The listing builds one solid part. Answer for the finished solid, in the listing's coordinates (mm). A direction names the side the tool comes from. Coordinates: 2 decimals unless noted, no trailing zeros. Write each loop counter-clockwise with the first axis right and the second up, starting at its lowest first coordinate (ties: lowest second). Pieces come first, ordered by that corner, then holes.
from build123d import *

# Parameters (mm, degrees)
SKETCH107_W         = 48
SKETCH107_H         = 56
PAD026_DEPTH        = 2
SKETCH108_R         = 1.75
HOLE046_DEPTH       = 25
SKETCH109_W         = 48
SKETCH109_H         = 32
PAD027_DEPTH        = 30
SKETCH110_W         = 40.4
SKETCH110_H         = 24.4
POCKET033_DEPTH     = 30
SKETCH111_W         = 20
SKETCH111_H         = 20
SKETCH111_W_2       = 40
POCKET034_DEPTH     = 28
SKETCH112_W         = 24
SKETCH112_H         = 22
POCKET035_DEPTH     = 50
SKETCH113_R         = 1.75
HOLE047_DEPTH       = 25
HOLE048_D           = 3.5
HOLE048_DEPTH       = 25
HOLE048_CSINK_D     = 8
HOLE048_CSINK_ANGLE = 90
HOLE048_TIPS_R      = 1.75
FILLET037_R         = 1
PAD_DEPTH           = 14
SKETCH115_R         = 4
HOLE_DEPTH          = 25
HOLE_TIPS_R         = 4
FILLET_R            = 1
FILLET038_R         = 1
FILLET039_R         = 1


with BuildPart() as part:
    # Sketch107 → Pad026 (new body)
    with BuildSketch(Plane.XY):
        Rectangle(SKETCH107_W, SKETCH107_H)
    extrude(amount=PAD026_DEPTH)

    # Sketch108 (on Face6 of Pad026) → Hole046 (cut)
    with BuildSketch(Plane.XY.offset(2)):
        with Locations((18, 22)):
            Circle(SKETCH108_R)
        with Locations((18, -22)):
            Circle(SKETCH108_R)
    hole046 = extrude(amount=-HOLE046_DEPTH, mode=Mode.SUBTRACT)

    # Mirrored041: Hole046 across Sketch108 V_Axis
    add(hole046.mirror(Plane(origin=(0, 0, 2), x_dir=(0, 0, 1), z_dir=(1, 0, 0))), mode=Mode.SUBTRACT)

    # Sketch109 (on Face5 of Mirrored041) → Pad027 (join)
    with BuildSketch(Plane.XY.offset(2)):
        Rectangle(SKETCH109_W, SKETCH109_H)
    extrude(amount=PAD027_DEPTH)

    # Sketch110 (on Face12 of Pad027) → Pocket033 (cut)
    with BuildSketch(Plane.XY.offset(32)):
        Rectangle(SKETCH110_W, SKETCH110_H)
    extrude(amount=-POCKET033_DEPTH, mode=Mode.SUBTRACT)

    # Sketch111 (on Face8 of Pocket033) → Pocket034 (cut)
    with BuildSketch(Plane.XY.offset(32)):
        with Locations((0, 10)):
            Rectangle(SKETCH111_W, SKETCH111_H)
        with Locations((20, 0)):
            Rectangle(SKETCH111_W_2, SKETCH111_H)
    extrude(amount=-POCKET034_DEPTH, mode=Mode.SUBTRACT)

    # Sketch112 (on Face3 of Pocket034) → Pocket035 (cut)
    with BuildSketch(Plane(origin=(-24, 0, 0), x_dir=(0, -1, 0), z_dir=(-1, 0, 0))):
        with Locations((0, 14)):
            Rectangle(SKETCH112_W, SKETCH112_H)
    extrude(amount=-POCKET035_DEPTH, mode=Mode.SUBTRACT)

    # Sketch113 (on Face34 of Pocket035) → Hole047 (cut)
    with BuildSketch(Plane.XY.offset(2)):
        with Locations((-16.2, 8.2)):
            Circle(SKETCH113_R)
        with Locations((-16.2, -8.2)):
            Circle(SKETCH113_R)
    extrude(amount=-HOLE047_DEPTH, mode=Mode.SUBTRACT)

    # Hole048
    with Locations(Plane(origin=(0, 0, 0), x_dir=(1, 0, 0), z_dir=(0, 0, -1))):
        with Locations((-16.2, -8.2), (-16.2, 8.2)):
            CounterSinkHole(HOLE048_D / 2, HOLE048_CSINK_D / 2, depth=HOLE048_DEPTH, counter_sink_angle=HOLE048_CSINK_ANGLE)

    # Hole048 tips → Hole048 tip 1 section 0
    with BuildSketch(Plane(origin=(0, 0, 25), x_dir=(1, 0, 0), z_dir=(0, 0, -1)), mode=Mode.PRIVATE) as hole048_tip_1_s0:
        with Locations((-16.2, -8.2)):
            Circle(HOLE048_TIPS_R)
    loft([hole048_tip_1_s0.sketch, Vertex(-16.2, 8.2, 26.051506)], mode=Mode.SUBTRACT)

    # Hole048 tips → Hole048 tip 2 section 0
    with BuildSketch(Plane(origin=(0, 0, 25), x_dir=(1, 0, 0), z_dir=(0, 0, -1)), mode=Mode.PRIVATE) as hole048_tip_2_s0:
        with Locations((-16.2, 8.2)):
            Circle(HOLE048_TIPS_R)
    loft([hole048_tip_2_s0.sketch, Vertex(-16.2, -8.2, 26.051506)], mode=Mode.SUBTRACT)

    # Fillet037
    fillet037_edges = [part.edges().sort_by_distance(p)[0] for p in [
        (24, -28, 1),
        (24, 28, 1),
        (-24, -28, 1),
        (-24, 28, 1),
    ]]
    fillet(fillet037_edges, radius=FILLET037_R)

    # Sketch (on Face10 of Fillet037) → Pad (join)
    with BuildSketch(Plane.YZ.offset(24)):
        with BuildLine():
            ThreePointArc((16, 12.999996), (19.221827, 5.221824), (27, 2))
            Line((16, 2), (27, 2))
            Line((16, 12.999996), (16, 2))
        make_face()
    pad = extrude(amount=-PAD_DEPTH)

    # Mirrored: Pad across Sketch V_Axis
    add(pad.mirror(Plane(origin=(24, 0, 0), x_dir=(1, 0, 0), z_dir=(0, 1, 0))))

    # Sketch115 (on Face5 of Pad) → Hole (cut)
    with BuildSketch(Plane.XY.offset(2)):
        with Locations((18, 22)):
            Circle(SKETCH115_R)
        with Locations((18, -22)):
            Circle(SKETCH115_R)
    extrude(amount=HOLE_DEPTH, mode=Mode.SUBTRACT)

    # Hole tips → Hole tip 1 section 0
    with BuildSketch(Plane.XY.offset(27), mode=Mode.PRIVATE) as hole_tip_1_s0:
        with Locations((18, 22)):
            Circle(HOLE_TIPS_R)
    loft([hole_tip_1_s0.sketch, Vertex(18, 22, 29.403442)], mode=Mode.SUBTRACT)

    # Hole tips → Hole tip 2 section 0
    with BuildSketch(Plane.XY.offset(27), mode=Mode.PRIVATE) as hole_tip_2_s0:
        with Locations((18, -22)):
            Circle(HOLE_TIPS_R)
    loft([hole_tip_2_s0.sketch, Vertex(18, -22, 29.403442)], mode=Mode.SUBTRACT)

    # Fillet
    fillet_edges = [part.edges().sort_by_distance(p)[0] for p in [
        (-24, -16, 17),
        (-24, 16, 17),
    ]]
    fillet(fillet_edges, radius=FILLET_R)

    # Fillet038
    fillet038_edges = [part.edges().sort_by_distance(p)[0] for p in [
        (20.2, 10, 28.5),
        (20.2, -10, 28.5),
    ]]
    fillet(fillet038_edges, radius=FILLET038_R)

    # Fillet039
    fillet039_edges = [part.edges().sort_by_distance(p)[0] for p in [
        (24, 10, 28.5),
        (24, -10, 28.5),
    ]]
    fillet(fillet039_edges, radius=FILLET039_R)


solid = part.part
1. Section B-B on y = 8.2 is taken. Give the vertices of the cut face in (x, z).
Results found:
outline: (-24, 0) - (-20.2, 0) - (-18.2, 2) - (-20.2, 2) - (-20.2, 3) - (-24, 3) - close; (-24, 25) - (-20.2, 25) - (-20.2, 32) - (-24, 32) - close; (-14.2, 2) - (-12.2, 0) - (24, 0) - (24, 3) - (20.2, 3) - (20.2, 2) - close
2. Find the intervals of material crossed by L1, parallel to Y at x = 18, z = 0.9; L2, parallel to Y at x = -18.5, z = 18; L3, parallel to X at y = 15, z = 28.5, in increasing order.
Results found:
L1: y = -28 to -23.75, -20.25 to 20.25, 23.75 to 28
L2: y = -16 to -12.2, 12.2 to 16
L3: x = -24 to -10, 10 to 24
3. Section A-A on z = 17 is taken. Give the vertices of the cut face in (x, y), then the cut area to 3 significant figures.
Results found:
outline: (-24, -15) arc R1 ccw to (-23, -16) - (24, -16) - (24, -12) - (20.2, -12) - (20.2, -12.2) - (-20.2, -12.2) - (-20.2, -12) - (-24, -12) - close; (-24, 12) - (-20.2, 12) - (-20.2, 12.2) - (-10, 12.2) - (-10, 16) - (-23, 16) arc R1 ccw to (-24, 15) - close; (10, 12.2) - (20.2, 12.2) - (20.2, 12) - (24, 12) - (24, 16) - (10, 16) - close
area: 291 mm2
4. Section D-D on y = 22 is taken. Give the vertices of the cut face in (x, z), then the cut area to 3 significant figures.
Results found:
outline: (-24, 0) - (-19.75, 0) - (-19.75, 2) - (-24, 2) - close; (-16.25, 0) - (16.25, 0) - (16.25, 2) - (14, 2) - (14, 3.2) - (10, 3.2) - (10, 2) - (-16.25, 2) - close; (19.75, 0) - (24, 0) - (24, 3.2) - (22, 3.2) - (22, 2) - (19.75, 2) - close
area: 89.2 mm2
5. Section C-C on x = 18 is taken. State how many separate pieces and enclosed holes the cut face has, then the cut area to 3 significant figures.
Results found:
separate pieces: 3
enclosed holes: 0
area: 353 mm2
6. A tool of negligible diameter and unlimited length cuts with its end or side. For faces 1 (the flat face through (10, 15, 16)), 2 (the flat face through (20, 21, 2)), 3 (the flat face through (22, 12, 14)), from which of +Z, -Z, +X, -X, +Y, -Y can it reach the whole face along a straight path? Write none if from no direction.
Results found:
face 1: +Z, +Y
face 2: +Z
face 3: +X, -X
7. Flat-ended cylindrical pins translate along their axes: P1, Ø2, axis at x = -18, y = 22, coming from the -Z side; P2, Ø14.5, axis at x = -8, y = 19.5, coming from the +Z side; P3, Ø1, axis at x = -2.5, z = 6.5, coming from the +Y side; P4, Ø1, axis at x = -0.5, y = -3, coming from the +Z side. Find the tip coordinate at first contact, or state that the pin passes through.
Results found:
P1: passes through
P2: stops at z = 32
P3: stops at y = -12.2
P4: stops at z = 2
8. For a pull along X with two mould halves and no side action, classify faces 4 (the flat face through (20, -23, 2)), 5 (the flat face through (24, 0, 2)), 6 (the flat face through (-24, -2.1, 25.4)) as pulls with the +X half, pulls with the -X half, needs draft (parallel to the pull), parting line crosses it, or undercut.
Results found:
face 4: undercut
face 5: pulls with the +X half
face 6: pulls with the -X half
